Can you work these out from the model? Positions are in its coordinate system, mm. Face numbers are marked on the shaded views. A direction names the side the tool comes from. Give positions to 0.01 mm unless a question says otherwise; leave off trailing zeros. Order: outer loops, then holes, each group sorted by start corner. A loop starts at its lowest first (then second) coordinate and runs counter-clockwise, first axis right, second up. Notation, with made-up numbers: M 34.25,81 L 93.25,81 A21 cw 93.25,111 Z; hole C 56,31 d8. An arc over 180 degrees is marked long. Use one line per item in the form item = value. Start each with the question number.
1. Will these pins go through, and if not, where does the flat tip stop? P1, Ø3, axis at x = 4, y = 10, coming from the -Z side; P2, Ø1, axis at x = -3.5, z = 10, coming from the +Y side; P3, Ø4, axis at y = 6.5, z = 0, coming from the +X side.
2. I need wall thicknesses on L1, parallel to Z at x = 0, y = 11.8; L2, parallel to Y at x = -7, z = 0; L3, parallel to Z at x = -2, y = 13.75. Which ranges of each line are inside material? Lowest first, please.
3. I want a section at A-A, the plane y = 3.75. List the corners of the cut face in (x, z) for me.
4. For the marked faces 1 and 2, which set-ups out of +Z, -Z, +X, -X, +Y, -Y let a thin tool reach every point of the face, with its end or its side?
5. I want a section at B-B, the plane z = 0. Count the separate pieces of the cut face and the enclosed holes in it, and give its area (3 significant figures).
6. We'd pull the mould along Z, two halves only. Please class the marked faces 3, 4 and 5: +Z half, -Z half, draft (parallel to the pull), parting line (faces both ways), or undercut.
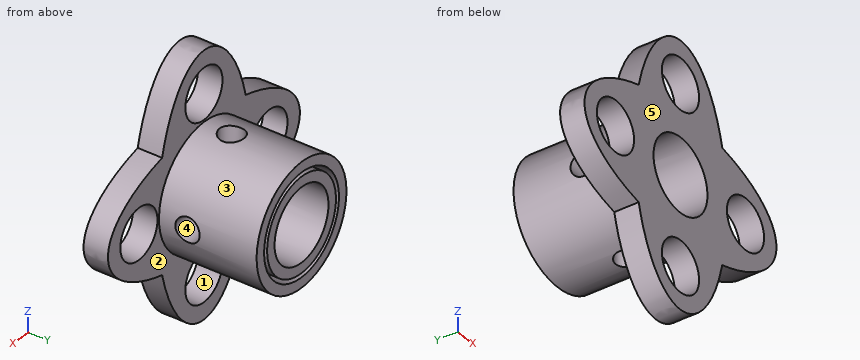
```python
from build123d import *

# Parameters (mm, degrees)
SKETCH1_R               = 3.1
SKETCH1_R_2             = 7.5
BOSS_EXTRUDE1_DEPTH     = 3
SKETCH1_3_R             = 7.5
SKETCH1_3_R_2           = 4.5
BOSS_EXTRUDE2_DEPTH     = 10
CUT_EXTRUDE1_DEPTH      = 25.762107606
CUT_EXTRUDE1_DEPTH_BACK = 25.762107606
SKETCH2_R               = 1.5
CUT_EXTRUDE2_DEPTH      = 25.762107646
CUT_EXTRUDE2_DEPTH_BACK = 25.762107646
SKETCH3_R               = 1.5
SKETCH29_R              = 7.5
SKETCH29_R_2            = 4.5
BOSS_EXTRUDE3_DEPTH     = 5
SKETCH30_R              = 6.25
SKETCH30_R_2            = 5.75
CUT_EXTRUDE_THIN1_DEPTH = 5


with BuildPart() as part:
    # Sketch1 → Boss-Extrude1 (new body)
    with BuildSketch(Plane(origin=(0, 0, 0), x_dir=(1, 0, 0), z_dir=(0, 1, 0))):
        with BuildLine():
            add(Edge.make_bspline(
                [(-6.976356378, -6.976356378), (0, -36.778651981), (6.976356378, -6.976356378)],
                knots=[5.16301411, 5.16301411, 5.16301411, 7.403356504, 7.403356504, 7.403356504], degree=2, weights=[1, 0.435528345, 1]))
            add(Edge.make_bspline(
                [(6.976356378, -6.976356378), (36.778651981, 0), (6.976356378, 6.976356378)],
                knots=[5.16301411, 5.16301411, 5.16301411, 7.403356504, 7.403356504, 7.403356504], degree=2, weights=[1, 0.435528345, 1]))
            add(Edge.make_bspline(
                [(6.976356378, 6.976356378), (0, 36.778651981), (-6.976356378, 6.976356378)],
                knots=[2.021421456, 2.021421456, 2.021421456, 4.261763851, 4.261763851, 4.261763851], degree=2, weights=[1, 0.435528345, 1]))
            add(Edge.make_bspline(
                [(-6.976356378, 6.976356378), (-36.778651981, 0), (-6.976356378, -6.976356378)],
                knots=[2.021421456, 2.021421456, 2.021421456, 4.261763851, 4.261763851, 4.261763851], degree=2, weights=[1, 0.435528345, 1]))
        make_face()
        with Locations(Location((-10.851478773, 0, 0), (0, 0, 270))):
            Circle(SKETCH1_R, mode=Mode.SUBTRACT)
        with Locations(Location((0, 10.851478773, 0), (0, 0, 270))):
            Circle(SKETCH1_R, mode=Mode.SUBTRACT)
        with Locations(Location((0, -10.851478773, 0), (0, 0, 270))):
            Circle(SKETCH1_R, mode=Mode.SUBTRACT)
        with Locations(Location((10.851478773, 0, 0), (0, 0, 270))):
            Circle(SKETCH1_R, mode=Mode.SUBTRACT)
        with Locations(Location((0, 0, 0), (0, 0, 270))):
            Circle(SKETCH1_R_2, mode=Mode.SUBTRACT)
    extrude(amount=BOSS_EXTRUDE1_DEPTH)

    # Sketch1_3 → Boss-Extrude2 (add)
    with BuildSketch(Plane(origin=(0, 0, 0), x_dir=(1, 0, 0), z_dir=(0, 1, 0))):
        with Locations(Location((0, 0, 0), (0, 0, 270))):
            Circle(SKETCH1_3_R)
        with Locations(Location((0, 0, 0), (0, 0, 270))):
            Circle(SKETCH1_3_R_2, mode=Mode.SUBTRACT)
    extrude(amount=BOSS_EXTRUDE2_DEPTH)

    # Sketch2 → Cut-Extrude1 (cut, two sides: drawn at the far end of the back side and taken through both)
    with BuildSketch(Plane.XY.offset(-CUT_EXTRUDE1_DEPTH_BACK)):
        with Locations((0, 6.432645923)):
            Circle(SKETCH2_R)
    extrude(amount=CUT_EXTRUDE1_DEPTH + CUT_EXTRUDE1_DEPTH_BACK, mode=Mode.SUBTRACT)

    # Sketch3 → Cut-Extrude2 (cut, two sides: drawn at the far end of the back side and taken through both)
    with BuildSketch(Plane(origin=(0, 0, 0), x_dir=(0, 0, -1), z_dir=(1, 0, 0)).offset(-CUT_EXTRUDE2_DEPTH_BACK)):
        with Locations((0, 6.5)):
            Circle(SKETCH3_R)
    extrude(amount=CUT_EXTRUDE2_DEPTH + CUT_EXTRUDE2_DEPTH_BACK, mode=Mode.SUBTRACT)

    # Sketch29 → Boss-Extrude3 (add)
    with BuildSketch(Plane(origin=(0, 10, 0), x_dir=(1, 0, 0), z_dir=(0, 1, 0))):
        with Locations(Location((0, 0, 0), (0, 0, 270))):
            Circle(SKETCH29_R)
        with Locations(Location((0, 0, 0), (0, 0, 270))):
            Circle(SKETCH29_R_2, mode=Mode.SUBTRACT)
    extrude(amount=BOSS_EXTRUDE3_DEPTH)

    # Sketch30 → Cut-Extrude-Thin1 (cut)
    with BuildSketch(Plane(origin=(0, 15, 0), x_dir=(1, 0, 0), z_dir=(0, 1, 0))):
        Circle(SKETCH30_R)
        Circle(SKETCH30_R_2, mode=Mode.SUBTRACT)
    extrude(amount=-CUT_EXTRUDE_THIN1_DEPTH, mode=Mode.SUBTRACT)


solid = part.part
```
Check result:
q1.P1 = -7.07
q1.P2 = 3
q1.P3 = 7.5
q2.L1 = -7.5 to -6.25, -5.75 to -4.5, 4.5 to 5.75, 6.25 to 7.5
q2.L2 = 0 to 5, 8 to 15
q2.L3 = -7.23 to -5.92, -5.39 to -4.03, 4.03 to 5.39, 5.92 to 7.23
q3.outline = C 0,0 d15; hole C 0,0 d9
q4.face_1 = +Y, -Y
q4.face_2 = +Y
q5.separate_pieces = 6
q5.enclosed_holes = 0
q5.area = 80.9 mm2
q6.face_3 = parting line
q6.face_4 = undercut
q6.face_5 = draft
